Here's the drawing with two shaded views (mm, measured from the low corner). I have some questions. Coordinates: 2 decimals unless noted, no trailing zeros. Loops run counter-clockwise (first coordinate to the right, second up) from the corner with the lowest first, then second, coordinate; pieces in that order, holes last.
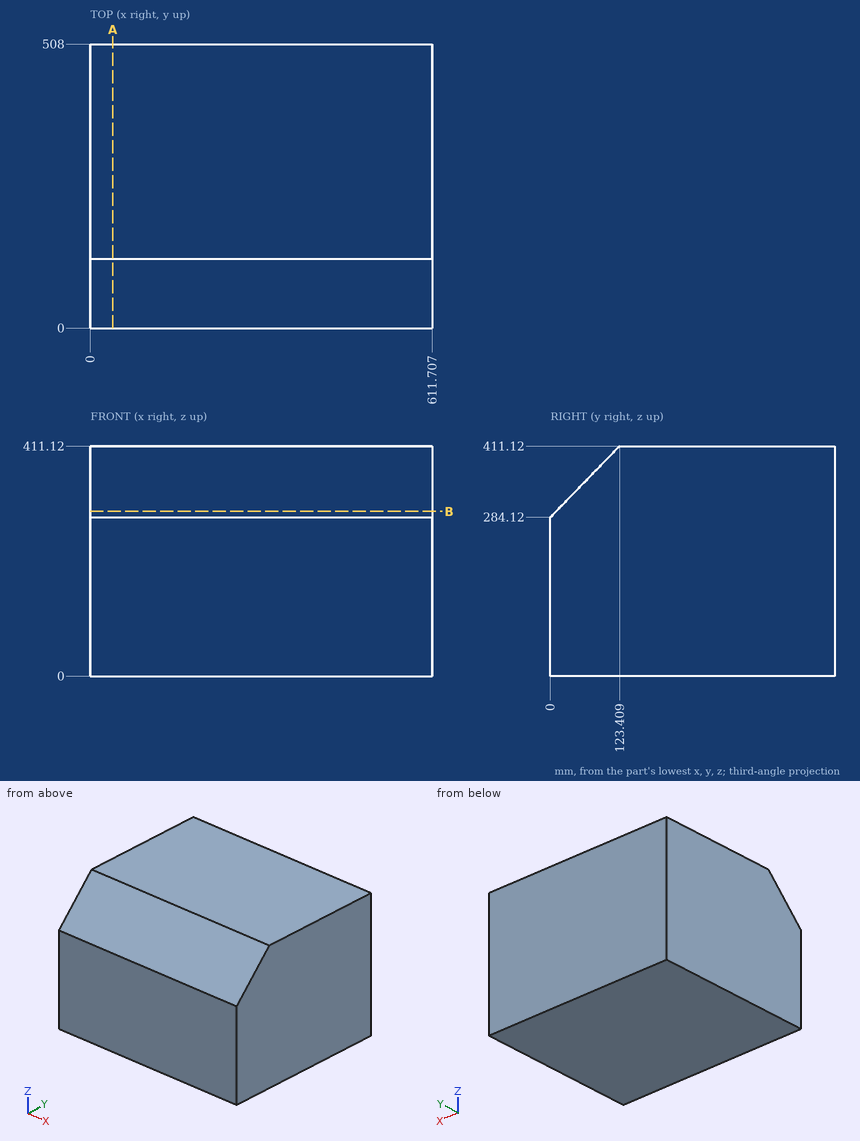
(1) If I drill on probe 1 along Y at (x, z) = (532, 343.5); probe 2 along Y at (x, z) = (182, 312); probe 3 along Z at (x, y) = (292, 118) (1 decimal), over which ranges is the centre line in solid material (lowest first)?
Check values:
probe 1: y = 57.7 to 508
probe 2: y = 27.09 to 508
probe 3: z = 0 to 405.6
(2) I'm going to push a flat-ended pin straight in: pin 1 (5 mm diameter, centred on x = 521.5, z = 76, fed in from -Y). Where does the tip first touch, or does it pass through?
Check values:
pin 1: stops at y = 0
(3) I want a section at A-A on x = 40. Write out the boundary of the cut face in (y, z).
Check values:
outline: (0, 0) - (508, 0) - (508, 411.12) - (123.41, 411.12) - (0, 284.12) - close
(4) I want a section at B-B on z = 294.5. Write out the boundary of the cut face in (x, y), then the cut area to 3 significant figures.
Check values:
outline: (0, 10.09) - (611.71, 10.09) - (611.71, 508) - (0, 508) - close
area: 305,000 mm2
